Verification items for the finished model (mm, model axes). Round coordinates to 2 decimals unless told otherwise and drop trailing zeros. Write each loop counter-clockwise with the first axis right and the second up, starting at its lowest first coordinate (ties: lowest second). Pieces come first, ordered by that corner, then holes. Notation, with made-up numbers: M -11.5,9 L 15.5,9 A19 ccw 15.5,23 Z; hole C 18.5,26 d6. An arc over 180 degrees is marked long. One line per item, written item: value. Start each with the question number.
Item 1: Thickness scan on probe 1 along Y at (x, z) = (0, 1.9); probe 2 along X at (y, z) = (-5.5, 0.75); probe 3 along X at (y, z) = (-88.25, 2.5). Record the ranges inside material, lowest first. Write a range as from..to.
Item 2: Gauge pin test, flat ends, axial feed: pin 1 (1.4 mm diameter, centred on y = 2.5, z = 2, fed in from -X); pin 2 (2.5 mm diameter, centred on x = 0, y = 88.25, fed in from -Z); pin 3 (1.7 mm diameter, centred on x = -94, z = 1, fed in from -Y); pin 4 (1.4 mm diameter, centred on y = 2, z = 2, fed in from +X). Record the tip position at first contact, or that the pin passes through.
Item 3: Section check A-A, the plane y = -29.5. Record the cut outline in (x, z).
Item 4: Section check B-B, the plane z = 2.1. State how many separate pieces and enclosed holes the cut face has, then the cut area to 3 significant figures.
Item 5: Section check C-C, the plane x = 83.5. Record the cut outline in (y, z).
from build123d import *

# Parameters (mm, degrees)
SKETCH2_W           = 206.36
SKETCH2_H           = 173.64
BOSS_EXTRUDE1_DEPTH = 3.18
CUT_EXTRUDE1_DEPTH  = 135.884903529
SKETCH9_W           = 10
SKETCH9_H           = 3.18
BOSS_EXTRUDE4_DEPTH = 3.18
SKETCH11_R          = 1.47
CUT_EXTRUDE3_DEPTH  = 137.953367246
SKETCH12_W          = 96
SKETCH12_H          = 66
CUT_EXTRUDE4_DEPTH  = 137.953367246


with BuildPart() as part:
    # Sketch2 → Boss-Extrude1 (new body)
    with BuildSketch(Plane.XY):
        Rectangle(SKETCH2_W, SKETCH2_H)
    extrude(amount=BOSS_EXTRUDE1_DEPTH)

    # Sketch3 → Cut-Extrude1 (cut, through all)
    with BuildSketch(Plane.XY.offset(3.18)):
        Polygon((-95.32, -1.47), (-95.32, -3.25), (-97.92, -3.25), (-97.92, -1.47), (-100, -1.47), (-100, -5), (-103.18, -5), (-103.18, 5), (-100, 5), (-100, 1.47), (-97.92, 1.47), (-97.92, 3.25), (-95.32, 3.25), (-95.32, 1.47), (-93.25, 1.47), (-93.25, -1.47), align=None)
    cut_extrude1 = extrude(amount=-CUT_EXTRUDE1_DEPTH, mode=Mode.SUBTRACT)

    # Sketch9 → Boss-Extrude4 (add)
    with BuildSketch(Plane(origin=(0, 86.82, 0), x_dir=(1, 0, 0), z_dir=(0, 1, 0))):
        with Locations((0, -1.59)):
            Rectangle(SKETCH9_W, SKETCH9_H)
    boss_extrude4 = extrude(amount=BOSS_EXTRUDE4_DEPTH)

    # Sketch11 → Cut-Extrude3 (cut, through all)
    with BuildSketch(Plane.XY.offset(3.18)):
        with Locations((0, 88.25)):
            Circle(SKETCH11_R)
    cut_extrude3 = extrude(amount=-CUT_EXTRUDE3_DEPTH, mode=Mode.SUBTRACT)

    # Mirror1: Cut-Extrude1 across plane
    add(cut_extrude1.mirror(Plane(origin=(0, 0, 0), x_dir=(0, 0, 1), z_dir=(1, 0, 0))), mode=Mode.SUBTRACT)

    # Mirror2: Boss-Extrude4, Cut-Extrude3 across plane
    add(boss_extrude4.mirror(Plane.ZX))
    add(cut_extrude3.mirror(Plane.ZX), mode=Mode.SUBTRACT)

    # Sketch12 → Cut-Extrude4 (cut, through all)
    with BuildSketch(Plane.XY.offset(3.18)):
        Rectangle(SKETCH12_W, SKETCH12_H)
    extrude(amount=-CUT_EXTRUDE4_DEPTH, mode=Mode.SUBTRACT)


solid = part.part
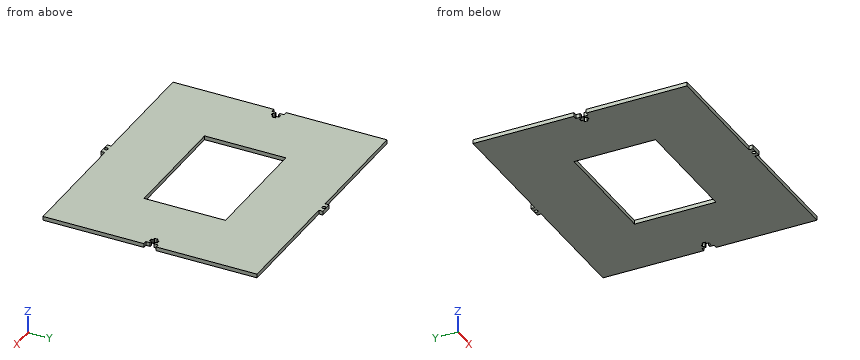
Response values:
1. probe 1: y = -90..-89.72, -86.78..-33, 33..86.78, 89.72..90
1. probe 2: x = -103.18..-48, 48..103.18
1. probe 3: x = -5..-1.47, 1.47..5
2. pin 1: stops at x = -100
2. pin 2: passes through
2. pin 3: stops at y = -86.82
2. pin 4: stops at x = 100
3. outline: M -103.18,0 L -48,0 L -48,3.18 L -103.18,3.18 Z; M 48,0 L 103.18,0 L 103.18,3.18 L 48,3.18 Z
4. separate pieces: 1
4. enclosed holes: 3
4. area: 29,400 mm2
5. outline: M -86.82,0 L 86.82,0 L 86.82,3.18 L -86.82,3.18 Z
